The listing builds one solid part. Answer for the finished solid, in the listing's coordinates (mm). A direction names the side the tool comes from. Give positions to 0.01 mm unless a question says otherwise; leave off trailing zeros. Loops run counter-clockwise (first coordinate to the right, second up) from the corner with the lowest first, then second, coordinate; pieces in that order, holes last. Notation, with made-up numbers: (78, -14) - (113, -14) arc R11 cw to (113, 6) - close; hole circle Ø11 at (63.25, -34.75). An arc over 180 degrees is marked (long way). Answer in a Markdown table with one row per item. Add a question column.
```python
from build123d import *

# Parameters (mm, degrees)
F0_R     = 2.5
F1_DEPTH = 37.4
F2_R     = 2
F3_R     = 1.825
F4_DEPTH = 4.8


with BuildPart() as f1:
    # F0 (on Top) → F1 (new body)
    with BuildSketch(Plane.XY):
        Circle(F0_R)
    extrude(amount=F1_DEPTH)

    # F2
    f2_edges = [f1.edges().sort_by_distance(p)[0] for p in [
        (-2.5, 0, 37.4),
    ]]
    fillet(f2_edges, radius=F2_R)

    # F3 (on face) → F4 (join)
    with BuildSketch(Plane(origin=(0, 0, 0), x_dir=(1, 0, 0), z_dir=(0, 0, -1))):
        Circle(F3_R)
    extrude(amount=F4_DEPTH)


solid = f1.part
```
(1) A tool of negligible diameter and unlimited length cuts with its end or side. For faces 1 (the face through (1.74, -0.55, -2.37)), 2 (the face through (0, 0, -4.8)), from which of +Z, -Z, +X, -X, +Y, -Y can it reach the whole face along a straight path? Write none if from no direction.
(2) A cutting plane is placed at A-A on z = -1.5. Determine the outline of the cut face in (x, y) (3 decimals).
(3) Given pin 1 Ø2 at (x, z) = (-1, 8.5) entering from +Y, flat-ended and moving along its own axis, determine where the tip first touches the part or whether it passes through.
(4) A cutting plane is placed at B-B on z = 25.5. Determine the outline of the cut face in (x, y), plus the area to 3 significant figures.
(5) Find the intervals of material crossed by line 1 along Y through (x, z) = (1.7, 9); line 2 along Y through (x, z) = (0.15, 13.5); line 3 along X through (y, z) = (-1.95, 18.5), in increasing order. Write a range as [from, to].
Evaluation:
| question | item | result |
|---|---|---|
| 1 | face 1 | -Z |
| 1 | face 2 | -Z, +X, -X, +Y, -Y |
| 2 | outline | circle Ø3.65 at (0, 0) |
| 3 | pin 1 | stops at y = 2.5 |
| 4 | outline | circle Ø5 at (0, 0) |
| 4 | area | 19.6 mm² |
| 5 | line 1 | y = [-1.83, 1.83] |
| 5 | line 2 | y = [-2.5, 2.5] |
| 5 | line 3 | x = [-1.56, 1.56] |
